The model under review builds one solid part; all positions refer to its coordinate system, in mm. Face numbers are marked on the shaded views. A direction names the side the tool comes from. Give positions to 0.01 mm unless a question says otherwise; leave off trailing zeros. Write each loop counter-clockwise with the first axis right and the second up, starting at its lowest first coordinate (ties: lowest second). Pieces come first, ordered by that corner, then holes. Notation, with made-up numbers: (63, 31.5) -> (100, 31.5) arc R10 cw to (100, 37.5) -> close; hole circle Ø3 at (69.25, -39). An arc over 180 degrees is marked (long way). Use CSV: the item, a comma, the result in double quotes.
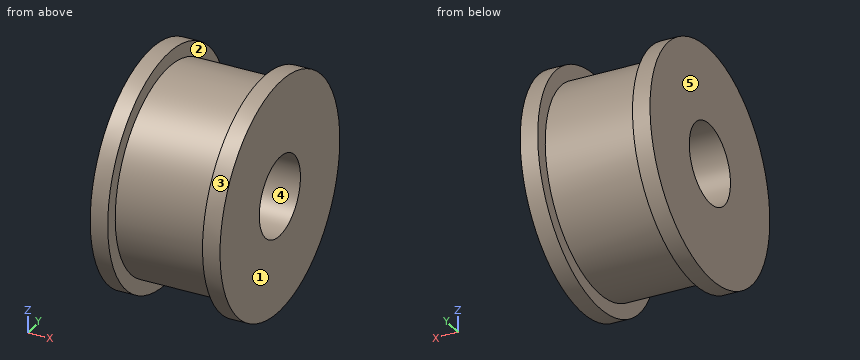
```python
from build123d import *

# Parameters (mm, degrees)
ESQUISSE2_R             = 27.5
ENL_V_MAT_EXTRU_1_DEPTH = 55


with BuildPart() as part:
    # Esquisse1 → Révolution2 (revolve)
    with BuildSketch(Plane(origin=(0, 0, 0), x_dir=(1, 0, 0), z_dir=(0, 1, 0))):
        Polygon((44.5, 0), (-44.5, 0), (-44.5, 80), (-32.5, 80), (-32.5, 70), (32.5, 70), (32.5, 80), (44.5, 80), align=None)
    revolve(axis=Axis((44.5, 0, 0), (-1, 0, 0)))

    # Esquisse2 → Enlèv. mat.-Extru.1 (cut, symmetric)
    with BuildSketch(Plane(origin=(0, 0, 0), x_dir=(0, 0, -1), z_dir=(1, 0, 0))):
        Circle(ESQUISSE2_R)
    extrude(amount=ENL_V_MAT_EXTRU_1_DEPTH, both=True, mode=Mode.SUBTRACT)


solid = part.part
```
Q1. Consider section A-A (y = 0). Write out the cut boundary in (x, z).
Derived:
outline,"(-44.5, -80) -> (-32.5, -80) -> (-32.5, -70) -> (32.5, -70) -> (32.5, -80) -> (44.5, -80) -> (44.5, -27.5) -> (-44.5, -27.5) -> close; (-44.5, 27.5) -> (44.5, 27.5) -> (44.5, 80) -> (32.5, 80) -> (32.5, 70) -> (-32.5, 70) -> (-32.5, 80) -> (-44.5, 80) -> close"
Q2. The part is to be moulded in two halves that separate along Z. For the marked faces 3, 4 and 5, say which applies: pulls with the +Z half, pulls with the -Z half, needs draft (parallel to the pull), parting line crosses it, or undercut.
Derived:
face 3,"parting line crosses it"
face 4,"undercut"
face 5,"needs draft"
Q3. Machinability: for the marked faces 1 and 2, which of the approach directions +Z, -Z, +X, -X, +Y, -Y give a long, thin tool a straight path to every point of the face, cutting with its end or side? Answer none if there is none.
Derived:
face 1,"+Z, -Z, +X, +Y, -Y"
face 2,"none"
Q4. Insertion check: pin 1 (12 mm diameter, centred on x = 23.5, y = 20.5, fed in from +Z); pin 2 (10 mm diameter, centred on x = 9, z = -36.5, fed in from -Y); pin 3 (8 mm diameter, centred on x = 2.5, z = -13, fed in from -Y). Each pin has a flat end and moves straight along its axis. Give the tip position at first contact, or say it passes through.
Derived:
pin 1,"stops at z = 68.48"
pin 2,"stops at y = -62.51"
pin 3,"stops at y = -69.42"
Q5. To check wall thickness, follow probe 1 along Y at (x, z) = (-4, 0); probe 2 along X at (y, z) = (-66, -25.5); probe 3 along Z at (x, y) = (-33.5, -3.5). State the ranges of each line that lie inside material, in increasing order.
Derived:
probe 1,"y = -70 to -27.5, 27.5 to 70"
probe 2,"x = -44.5 to -32.5, 32.5 to 44.5"
probe 3,"z = -79.92 to -27.28, 27.28 to 79.92"
Q6. Consider section D-D (z = -33.5). Write out the cut boundary in (x, y).
Derived:
outline,"(-44.5, -72.65) -> (-32.5, -72.65) -> (-32.5, -61.46) -> (32.5, -61.46) -> (32.5, -72.65) -> (44.5, -72.65) -> (44.5, 72.65) -> (32.5, 72.65) -> (32.5, 61.46) -> (-32.5, 61.46) -> (-32.5, 72.65) -> (-44.5, 72.65) -> close"
Q7. Consider section C-C (x = 6.5). Write out the cut boundary in (y, z).
Derived:
outline,"circle Ø140 at (0, 0); hole circle Ø55 at (0, 0)"
